```python
from build123d import *

# Parameters (mm, degrees)
ESQUISSE1_R             = 50
ESQUISSE1_R_2           = 11.75
BOSS_EXTRU_1_DEPTH      = 8
ESQUISSE2_R             = 1.6
ENL_V_MAT_EXTRU_1_DEPTH = 72.161787499
ESQUISSE3_R             = 2.85
ENL_V_MAT_EXTRU_2_DEPTH = 3


with BuildPart() as part:
    # Esquisse1 → Boss.-Extru.1 (new body)
    with BuildSketch(Plane.XY):
        Circle(ESQUISSE1_R)
        Circle(ESQUISSE1_R_2, mode=Mode.SUBTRACT)
    extrude(amount=-BOSS_EXTRU_1_DEPTH)

    # Esquisse2 → Enlèv. mat.-Extru.1 (cut, through all)
    with BuildSketch(Plane.XY):
        with Locations((30, 0)):
            Circle(ESQUISSE2_R)
        with Locations((-30, 0)):
            Circle(ESQUISSE2_R)
    extrude(amount=-ENL_V_MAT_EXTRU_1_DEPTH, mode=Mode.SUBTRACT)

    # Esquisse3 → Enlèv. mat.-Extru.2 (cut)
    with BuildSketch(Plane.XY):
        with Locations((30, 0)):
            Circle(ESQUISSE3_R)
        with Locations((-30, 0)):
            Circle(ESQUISSE3_R)
    extrude(amount=-ENL_V_MAT_EXTRU_2_DEPTH, mode=Mode.SUBTRACT)


solid = part.part
```
Geometry: final body of the model. Coordinates: model frame, mm. A direction names the side the tool comes from. Round coordinates to 2 decimals unless told otherwise and drop trailing zeros. Write each loop counter-clockwise with the first axis right and the second up, starting at its lowest first coordinate (ties: lowest second). Pieces come first, ordered by that corner, then holes.
Item 1: Material intervals for L1, parallel to Y at x = 0, z = -5.25; L2, parallel to X at y = -10.5, z = -1; L3, parallel to Y at x = 30, z = -6.3, sorted ascending.
Item 2: Set-up query: faces 1 (the face through (28.4, 0.07, -5.46)), 2 (the face through (-28, 0, -3)). Return all of +Z, -Z, +X, -X, +Y, -Y with unobstructed straight access to the full face (end or side cutting, diameter ignored); none if empty.
Item 3: Section query A-A (x = 0). Return loops of the section in (y, z).
Item 4: Mould query, pull axis Y, two halves, no side actions, for faces 3 (the face through (-12, 1, 0)), 4 (the face through (-27.367, -1.092, -1.479)), 5 (the face through (47.69, 15.02, -3.94)). Classes: +Y half, -Y half, draft (parallel to the pull), parting line (faces both ways), or undercut.
Item 5: Pin query (flat end, axial travel): P1, Ø3.5, axis at x = 30, y = 0, coming from the +Z side; P2, Ø4, axis at x = -37, y = -16.5, coming from the +Z side; P3, Ø4, axis at x = 36.5, z = -3.5, coming from the -Y side; P4, Ø4, axis at x = 17.5, z = -3, coming from the +Y side. Return the tip coordinate at first contact, or that it passes through.
Item 6: Section query C-C (x = -30). Return loops of the section in (y, z), plus the area to 3 significant figures.
Item 7: Section query D-D (z = -1.25). Return loops of the section in (x, y), plus the area to 3 significant figures.
Item 8: Section query B-B (y = 0). Return loops of the section in (x, z).
Completed:
1. L1: y = -50 to -11.75, 11.75 to 50
1. L2: x = -48.89 to -5.27, 5.27 to 48.89
1. L3: y = -40 to -1.6, 1.6 to 40
2. face 1: +Z, -Z
2. face 2: +Z
3. outline: (-50, -8) - (-11.75, -8) - (-11.75, 0) - (-50, 0) - close; (11.75, -8) - (50, -8) - (50, 0) - (11.75, 0) - close
4. face 3: draft
4. face 4: undercut
4. face 5: parting line
5. P1: stops at z = -3
5. P2: stops at z = 0
5. P3: stops at y = -36.19
5. P4: stops at y = 47.54
6. outline: (-40, -8) - (-1.6, -8) - (-1.6, -3) - (-2.85, -3) - (-2.85, 0) - (-40, 0) - close; (1.6, -8) - (40, -8) - (40, 0) - (2.85, 0) - (2.85, -3) - (1.6, -3) - close
6. area: 607 mm2
7. outline: circle Ø100 at (0, 0); hole circle Ø5.7 at (-30, 0); hole circle Ø23.5 at (0, 0); hole circle Ø5.7 at (30, 0)
7. area: 7,370 mm2
8. outline: (-50, -8) - (-31.6, -8) - (-31.6, -3) - (-32.85, -3) - (-32.85, 0) - (-50, 0) - close; (-28.4, -8) - (-11.75, -8) - (-11.75, 0) - (-27.15, 0) - (-27.15, -3) - (-28.4, -3) - close; (11.75, -8) - (28.4, -8) - (28.4, -3) - (27.15, -3) - (27.15, 0) - (11.75, 0) - close; (31.6, -8) - (50, -8) - (50, 0) - (32.85, 0) - (32.85, -3) - (31.6, -3) - close
